Here's how the part is built. I have some questions about the finished solid (model axes, mm). A direction names the side the tool comes from. Give positions to 0.01 mm unless a question says otherwise; leave off trailing zeros. Loops run counter-clockwise (first coordinate to the right, second up) from the corner with the lowest first, then second, coordinate; pieces in that order, holes last. Notation, with made-up numbers: (35, 11) -> (86, 11) arc R11 ccw to (86, 32) -> close; hole circle Ø5 at (3.25, 61.25). An arc over 180 degrees is marked (long way). Answer in a Markdown table with one row per item. Add a question column.
Item 1: Which directions (+Z, -Z, +X, -X, +Y, -Y) give clear straight access to the entire face, cutting with the end or side of a thin tool? Please do faces 5 (the face through (0, -10, -1)), 6 (the face through (1, 0, -3)), 7 (the face through (12, -21, 0)).
Item 2: If we section it at A-A (y = 3): Write out the boundary of the cut face in (x, z), then the cut area to 3 significant figures.
Item 3: For P1, Ø0.8, axis at x = 4, z = 0.5, coming from the -Y side; P2, Ø1.4, axis at x = 0.5, z = -3, coming from the +Y side; P3, Ø1.5, axis at x = 2.5, z = -3.5, coming from the -Y side, each with a flat end and sliding along its axis, tell me the tip position at first contact or that it passes through.
Item 4: If we section it at B-B (z = -0.5): Write out the boundary of the cut face in (x, y).
Item 5: If I drill on line 1 (X direction, y = -17, z = -3.5); line 2 (Z direction, x = 6.25, y = 0); line 3 (Y direction, x = 12.25, z = -2.75), over which ranges is the centre line in solid material (lowest first)?
Item 6: If we section it at C-C (x = 6.5): Write out the boundary of the cut face in (y, z).
Item 7: If we section it at D-D (z = 1.5): Write out the boundary of the cut face in (x, y), then the cut area to 3 significant figures.
Item 8: We'd pull the mould along Y, two halves only. Please class faces 1 (the face through (5.763, 3.676, 1.622)), 2 (the face through (6, 6, 2)), 3 (the face through (1, -13, -6)), 4 (the face through (0.62, -25.35, -0.08)): released by +Y, released by -Y, zero draft, split by the parting line, or undercut.
```python
from build123d import *

# Parameters (mm, degrees)
F1_DEPTH  = 13
F2_R      = 1
F3_DEPTH  = 9.201
F4_W      = 10.5
F4_H      = 6
F5_DEPTH  = 32.001
F6_R      = 1.5
F7_DEPTH  = 1.5
F8_R      = 1.4
F9_R      = 1.5
F10_DEPTH = 1.5
F11_R     = 1.4
F13_DEPTH = 13.001


with BuildPart() as f1:
    # F0 (on Right) → F1 (new body)
    with BuildSketch(Plane.YZ):
        Polygon((0, -6), (0, 0), (-17, 0), (-26, 0), (-26, -6), align=None)
        Polygon((-17, 0), (0, 0), (6, 0), (6, 3.2), (0, 3.2), (-17, 1), align=None)
    extrude(amount=F1_DEPTH)

    # F2 (on face) → F3 (cut, through all)
    with BuildSketch(Plane.XY.offset(3.2)):
        with Locations((6.5, 3.0000000261)):
            Circle(F2_R)
    extrude(amount=-F3_DEPTH, mode=Mode.SUBTRACT)

    # F4 (on face) → F5 (cut, through all)
    with BuildSketch(Plane.XZ.offset(26)):
        with Locations((6.5, -3)):
            Rectangle(F4_W, F4_H)
    extrude(amount=-F5_DEPTH, mode=Mode.SUBTRACT)

    # F6 (on face) → F7 (join)
    with BuildSketch(Plane.YZ.offset(1.25)):
        with Locations((-23.5, -3)):
            Circle(F6_R)
    extrude(amount=F7_DEPTH)

    # F8
    f8_edges = [f1.edges().sort_by_distance(p)[0] for p in [
        (2.75, -25, -3),
    ]]
    fillet(f8_edges, radius=F8_R)

    # F9 (on face) → F10 (join)
    with BuildSketch(Plane(origin=(11.75, 0, 0), x_dir=(0, -1, 0), z_dir=(-1, 0, 0))):
        with Locations((23.5, -3)):
            Circle(F9_R)
    extrude(amount=F10_DEPTH)

    # F11
    f11_edges = [f1.edges().sort_by_distance(p)[0] for p in [
        (10.25, -22, -3),
    ]]
    fillet(f11_edges, radius=F11_R)

    # F12 (on face) → F13 (cut, through all)
    with BuildSketch(Plane(origin=(0, 0, 0), x_dir=(0, -1, 0), z_dir=(-1, 0, 0))):
        Polygon((26, 0), (24.7272727273, 0), (26, -0.1647058824), align=None)
    extrude(amount=-F13_DEPTH, mode=Mode.SUBTRACT)


solid = f1.part
```
Recorded:
| question | item | result |
|---|---|---|
| 1 | face 5 | +Z, -Z, -X, +Y, -Y |
| 1 | face 6 | -Z, +X, -X, +Y |
| 1 | face 7 | +Z, +X, -X, -Y |
| 2 | outline | (0, 0) -> (5.5, 0) -> (5.5, 3.2) -> (0, 3.2) -> close; (7.5, 0) -> (13, 0) -> (13, 3.2) -> (7.5, 3.2) -> close |
| 2 | area | 35.2 mm^2 |
| 3 | P1 | stops at y = -17 |
| 3 | P2 | stops at y = 0 |
| 3 | P3 | stops at y = -24.91 |
| 4 | outline | (0, -26) -> (1.25, -26) -> (1.25, 0) -> (0, 0) -> close; (11.75, -26) -> (13, -26) -> (13, 0) -> (11.75, 0) -> close |
| 5 | line 1 | x = 0 to 1.25, 11.75 to 13 |
| 5 | line 2 | z = 0 to 3.2 |
| 5 | line 3 | y = -26 to 0 |
| 6 | outline | (-17, 0) -> (2, 0) -> (2, 3.2) -> (0, 3.2) -> (-17, 1) -> close; (4, 0) -> (6, 0) -> (6, 3.2) -> (4, 3.2) -> close |
| 7 | outline | (0, -13.14) -> (13, -13.14) -> (13, 6) -> (0, 6) -> close; hole circle Ø2 at (6.5, 3) |
| 7 | area | 246 mm^2 |
| 8 | face 1 | undercut |
| 8 | face 2 | released by +Y |
| 8 | face 3 | zero draft |
| 8 | face 4 | released by -Y |
